from build123d import *

# Parameters (mm, degrees)
BXBXS_8639_82_40_X_40_X_2_5_1_DEPTH = 2000


with BuildPart() as part:
    # Sketch1 → Труба bxbxs гост8639-82 40 X 40 X 2.5(1) (new body)
    with BuildSketch(Plane.YZ.offset(-1000)):
        with BuildLine():
            Line((-16.25, -20), (16.25, -20))
            ThreePointArc((16.25, -20), (18.901650429, -18.901650429), (20, -16.25))
            Line((20, -16.25), (20, 16.25))
            ThreePointArc((20, 16.25), (18.901650429, 18.901650429), (16.25, 20))
            Line((16.25, 20), (-16.25, 20))
            ThreePointArc((-16.25, 20), (-18.901650429, 18.901650429), (-20, 16.25))
            Line((-20, 16.25), (-20, -16.25))
            ThreePointArc((-20, -16.25), (-18.901650429, -18.901650429), (-16.25, -20))
        make_face()
        with BuildLine():
            Line((-16.25, -17.5), (16.25, -17.5))
            ThreePointArc((16.25, -17.5), (17.133883476, -17.133883476), (17.5, -16.25))
            Line((17.5, -16.25), (17.5, 16.25))
            ThreePointArc((17.5, 16.25), (17.133883476, 17.133883476), (16.25, 17.5))
            Line((16.25, 17.5), (-16.25, 17.5))
            ThreePointArc((-16.25, 17.5), (-17.133883476, 17.133883476), (-17.5, 16.25))
            Line((-17.5, 16.25), (-17.5, -16.25))
            ThreePointArc((-17.5, -16.25), (-17.133883476, -17.133883476), (-16.25, -17.5))
        make_face(mode=Mode.SUBTRACT)
    extrude(amount=BXBXS_8639_82_40_X_40_X_2_5_1_DEPTH)


solid = part.part
Work out the finished part from the listing and answer in its coordinate system (mm). A direction names the side the tool comes from. Give positions to 0.01 mm unless a question says otherwise; leave off trailing zeros. Loops run counter-clockwise (first coordinate to the right, second up) from the corner with the lowest first, then second, coordinate; pieces in that order, holes last. Notation, with made-up numbers: (78, 81.25) -> (113, 81.25) arc R34 cw to (113, 117.25) -> close; hole circle Ø1 at (83.5, -13.75). An arc over 180 degrees is marked (long way). Use a Markdown table: item, result. Add a question column.
1) Which of the six approach directions +Z, -Z, +X, -X, +Y, -Y give full straight-line access (tool end or side, diameter ignored) to faces 4 (the flat face through (-14, 0, -20)), 5 (the flat face through (-14, 17.5, 0))?
2) The part is cut by section A-A, the plane z = 8. Determine the outline of the cut face in (x, y).
3) Consider line 1 along Y through (x, z) = (294, 6.5). Determine where the line is inside the solid, lowest interval first.
4) For a pull along Y with two mould halves and no side action, classify faces 1 (the flat face through (-14, 20, 0)), 2 (the flat face through (-14, 0, 17.5)), 3 (the flat face through (-1000, -18, 2)) as +Y half, -Y half, draft (parallel to the pull), parting line (faces both ways), or undercut.
5) The part is cut by section C-C, the plane x = 873. Determine the outline of the cut face in (y, z).
Reported:
| question | item | result |
|---|---|---|
| 1 | face 4 | -Z, +X, -X, +Y, -Y |
| 1 | face 5 | +X, -X |
| 2 | outline | (-1000, -20) -> (1000, -20) -> (1000, -17.5) -> (-1000, -17.5) -> close; (-1000, 17.5) -> (1000, 17.5) -> (1000, 20) -> (-1000, 20) -> close |
| 3 | line 1 | y = -20 to -17.5, 17.5 to 20 |
| 4 | face 1 | +Y half |
| 4 | face 2 | undercut |
| 4 | face 3 | draft |
| 5 | outline | (-20, -16.25) arc R3.75 ccw to (-16.25, -20) -> (16.25, -20) arc R3.75 ccw to (20, -16.25) -> (20, 16.25) arc R3.75 ccw to (16.25, 20) -> (-16.25, 20) arc R3.75 ccw to (-20, 16.25) -> close; hole (-17.5, -16.25) arc R1.25 ccw to (-16.25, -17.5) -> (16.25, -17.5) arc R1.25 ccw to (17.5, -16.25) -> (17.5, 16.25) arc R1.25 ccw to (16.25, 17.5) -> (-16.25, 17.5) arc R1.25 ccw to (-17.5, 16.25) -> close |
